from build123d import *

# Parameters (mm, degrees)
F0_W      = 4.5
F0_H      = 20
F1_DEPTH  = 4
F2_W      = 5.5
F2_H      = 20
F3_DEPTH  = 2
F4_W      = 5
F4_H      = 5
F5_DEPTH  = 150
F6_W      = 5
F6_H      = 10
F7_DEPTH  = 10
F8_W      = 9.5
F8_H      = 16
F9_DEPTH  = 20
F10_W     = 15.690336
F10_H     = 16
F11_DEPTH = 30
F13_DEPTH = 16
F15_DEPTH = 5.5
F17_DEPTH = 4


with BuildPart() as f1:
    # F0 (on Top) → F1 (new body)
    with BuildSketch(Plane.XY):
        with Locations((2.25, 10)):
            Rectangle(F0_W, F0_H)
    extrude(amount=F1_DEPTH)

    # F2 (on Top) → F3 (join)
    with BuildSketch(Plane.XY):
        with Locations((7.25, 10)):
            Rectangle(F2_W, F2_H)
    extrude(amount=F3_DEPTH)

    # F4 (on Top) → F5 (join)
    with BuildSketch(Plane.XY):
        with Locations((12.5, 17.5)):
            Rectangle(F4_W, F4_H)
        Polygon((20, 20), (15, 20), (15, 15), (15, 5), (15, 0), (20, 0), align=None)
        Polygon((25.3, 20), (20, 20), (20, 0), align=None)
        with Locations((12.5, 2.5)):
            Rectangle(F4_W, F4_H)
    extrude(amount=F5_DEPTH)

    # F6 (on Top) → F7 (join)
    with BuildSketch(Plane.XY):
        with Locations((12.5, 10)):
            Rectangle(F6_W, F6_H)
    extrude(amount=F7_DEPTH)

    # F8 (on face) → F9 (join)
    with BuildSketch(Plane(origin=(18.687659, -4.95223, 0), x_dir=(0.256158, 0.966635, 0), z_dir=(0.966635, -0.256158, 0))):
        with Locations((16.063501, 8)):
            Rectangle(F8_W, F8_H)
        Polygon((20.813501, 16), (20.813501, 0), (25.813501, 0), (25.813501, 163), (20.813501, 163), align=None)
        Polygon((5.123165, 0), (11.313501, 0), (11.313501, 16), (11.313501, 150), (5.123165, 150), align=None)
    extrude(amount=F9_DEPTH)

    # F10 (on face) → F11 (join)
    with BuildSketch(Plane(origin=(38.020356, -10.075394, 0), x_dir=(0.256158, 0.966635, 0), z_dir=(0.966635, -0.256158, 0))):
        Polygon((25.813501, 0), (25.813501, 163), (20.813501, 163), (20.813501, 16), (20.813501, 0), align=None)
        with Locations((12.968333, 8)):
            Rectangle(F10_W, F10_H)
    extrude(amount=F11_DEPTH)

    # F12 (on face) → F13 (cut)
    with BuildSketch(Plane.XY.offset(16)):
        Polygon((72.350952, 2.358914), (39.332697, -5.123165), (68.331743, -12.807912), align=None)
    extrude(amount=-F13_DEPTH, mode=Mode.SUBTRACT)

    # F14 (on face) → F15 (join)
    with BuildSketch(Plane.XY.offset(163)):
        Polygon((24.531525, 17.100095), (24.019209, 15.166826), (72.350952, 2.358914), (72.863268, 4.292183), align=None)
    extrude(amount=F15_DEPTH)

    # F16 (on face) → F17 (join)
    with BuildSketch(Plane.XY.offset(168.5)):
        Polygon((24.787684, 18.06673), (24.019209, 15.166826), (72.350952, 2.358914), (73.119427, 5.258818), align=None)
    extrude(amount=F17_DEPTH)


solid = f1.part
Input: part model. Units: mm. Frame: model coordinates. A direction names the side the tool comes from. Give positions to 0.01 mm unless a question says otherwise; leave off trailing zeros. Write each loop counter-clockwise with the first axis right and the second up, starting at its lowest first coordinate (ties: lowest second). Pieces come first, ordered by that corner, then holes. Notation, with made-up numbers: M 78,65.5 L 98,65.5 A19 ccw 98,74.5 Z; hole C 55.5,-36 d3. An arc over 180 degrees is marked long. Write item = value, one per line. Start each with the question number.
1) Cut plane C-C on y = -3.25. Return the cut outline in (x, z).
2) Reachability of faces 1 (the flat face through (24.4, 16.6, 170.5)), 2 (the flat face through (7, 10, 2)), 3 (the flat face through (49.036, 10.606, 165.712)), 4 (the flat face through (31.117, 3.458, 82.062)), 5 (the flat face through (57.648, 6.255, 90.529)) from +Z, -Z, +X, -X, +Y, -Y: full face, straight path, thin tool, end or side. Return the list, or none.
3) First-contact query: pin 1 Ø3 at (x, y) = (58, -1.5) entering from +Z; pin 2 Ø5 at (y, z) = (8, 51.5) entering from -X; pin 3 Ø6 at (x, y) = (18.5, 3) entering from -Z; pin 4 Ø10 at (x, z) = (9, 89.5) entering from -Y. Flat tips, straight axial feed; report the tip coordinate or a pass-through.
4) Material intervals for line 1 along Z through (x, y) = (48, 11); line 2 along Z through (x, y) = (38, 11); line 3 along Z through (x, y) = (44, 14.5), sorted ascending. Write a range as [from, to].
5) Draft query along X for faces 6 (the flat face through (18, 20, 74)), 7 (the flat face through (33.55, 12.64, 90.53)), 8 (the flat face through (0, 10, 2)). Return one class per face: +X half, -X half, draft (parallel to the pull), parting line (faces both ways), or undercut.
Solved:
q1.outline = M 32.26,0 L 47.6,0 L 47.6,16 L 39.83,16 L 39.83,150 L 32.26,150 Z
q2.face_1 = +Z, -X, +Y
q2.face_2 = +Z, +Y, -Y
q2.face_3 = +X, +Y
q2.face_4 = +Z
q2.face_5 = +Z, -Y
q3.pin_1 = 16
q3.pin_2 = 15
q3.pin_3 = 0
q3.pin_4 = 0
q4.line_1 = [0, 163], [168.5, 172.5]
q4.line_2 = [0, 16]
q4.line_3 = [0, 163]
q5.face_6 = draft
q5.face_7 = undercut
q5.face_8 = -X half
